Verification items for this drawing (mm, ordinates from the low corner). A direction names the side the tool comes from. Coordinates: 2 decimals unless noted, no trailing zeros. Order: outer loops, then holes, each group sorted by start corner. A loop starts at its lowest first (then second) coordinate and runs counter-clockwise, first axis right, second up.
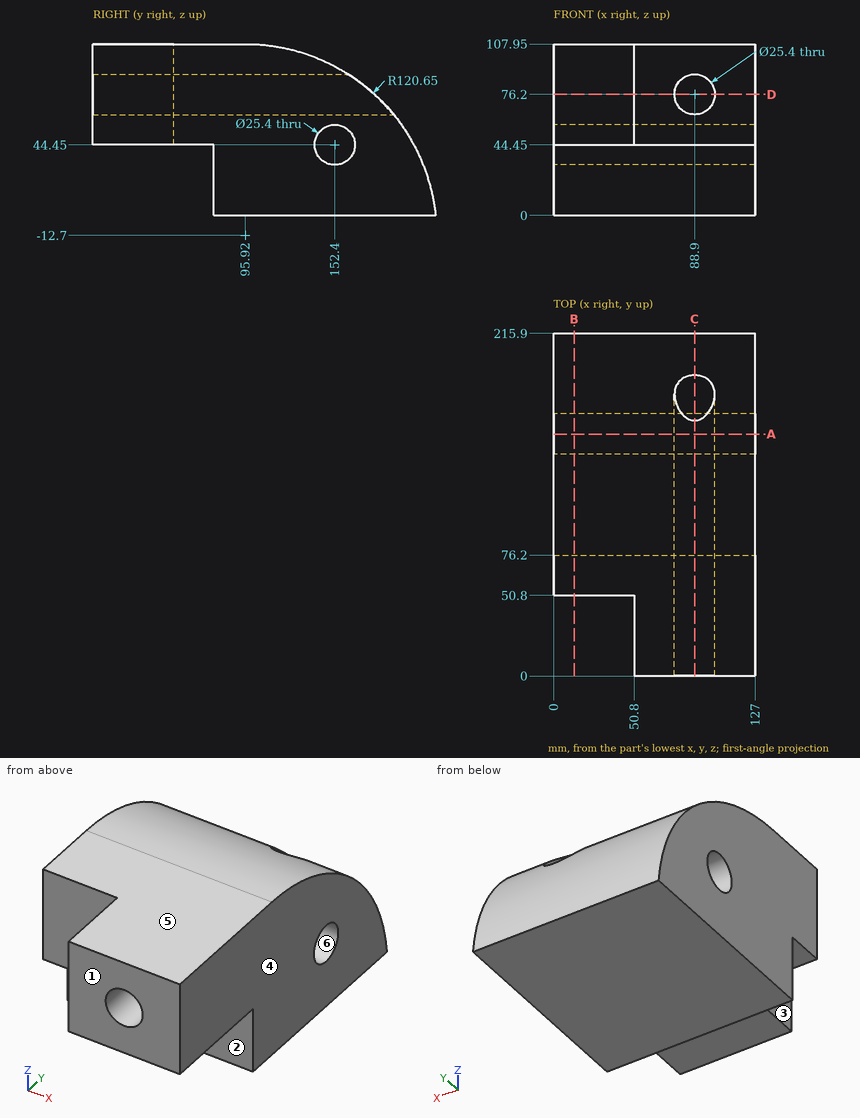
(1) Tool access check on the marked faces 1, 2 and 3. Record the directions out of +Z, -Z, +X, -X, +Y, -Y that give a thin tool (end or side, any length) a straight path to the whole face; none if there is none.
Filled in:
face 1: +Z, -Z, +X, -X, -Y
face 2: -Z, +X, -X, -Y
face 3: +Z, -Z, -X, -Y
(2) Cross-section at B-B (x = 13). Enter the section's corners in (y, z), and give its area (3 significant figures).
Filled in:
outline: (50.8, 44.45) - (76.2, 44.45) - (76.2, 0) - (215.9, 0) arc R120.65 ccw to (95.92, 107.95) - (50.8, 107.95) - close; hole circle Ø25.4 at (152.4, 44.45)
area: 13,100 mm2
(3) Cross-section at C-C (x = 88.9). Enter the section's corners in (y, z).
Filled in:
outline: (0, 44.45) - (76.2, 44.45) - (76.2, 0) - (215.9, 0) arc R120.65 ccw to (189.46, 63.5) - (0, 63.5) - close; (0, 88.9) - (160.99, 88.9) arc R120.65 ccw to (95.92, 107.95) - (0, 107.95) - close; hole circle Ø25.4 at (152.4, 44.45)
(4) Thickness scan on probe 1 along Z at (x, y) = (88.9, 41); probe 2 along Y at (x, z) = (36, 39.5) (1 decimal); probe 3 along Y at (x, z) = (116, 53). Record the ranges inside material, lowest first.
Filled in:
probe 1: z = 44.45 to 63.5, 88.9 to 107.95
probe 2: y = 76.2 to 140.7, 164.1 to 204.7
probe 3: y = 0 to 143.01, 161.79 to 197.11
(5) Release check for a two-part mould opening along Z. For the marked faces 4, 5 and 6 record: +Z half, -Z half, draft (parallel to the pull), parting line (faces both ways), or undercut.
Filled in:
face 4: draft
face 5: +Z half
face 6: undercut
(6) Go/stop test with flat-tipped pins: P1, Ø8, axis at x = 13, z = 78.5, coming from the +Y side; P2, Ø23, axis at x = 57.5, y = 45.5, coming from the -Z side; P3, Ø3, axis at x = 74.5, y = 177.5, coming from the +Z side. Record where each tip stops, or that it passes through.
Filled in:
P1: stops at y = 179.3
P2: stops at z = 44.45
P3: stops at z = 77.54
(7) Cross-section at A-A (y = 152.4). Enter the section's corners in (x, z), and give its area (3 significant figures).
Filled in:
outline: (0, 0) - (127, 0) - (127, 31.75) - (0, 31.75) - close; (0, 57.15) - (127, 57.15) - (127, 93.91) - (0, 93.91) - close; hole circle Ø25.4 at (88.9, 76.2)
area: 8,190 mm2
(8) Cross-section at D-D (z = 76.2). Enter the section's corners in (x, y), and give its area (3 significant figures).
Filled in:
outline: (0, 50.8) - (50.8, 50.8) - (50.8, 0) - (76.2, 0) - (76.2, 177.49) - (0, 177.49) - close; (101.6, 0) - (127, 0) - (127, 177.49) - (101.6, 177.49) - close
area: 15,500 mm2
